from build123d import *

# Parameters (mm, degrees)
BOSS_EXTRUDE1_DEPTH = 88.9
CUT_EXTRUDE1_DEPTH  = 102.108


with BuildPart() as part:
    # Sketch2 → Boss-Extrude1 (new body)
    with BuildSketch(Plane(origin=(0, 0, 0), x_dir=(1, 0, 0), z_dir=(0, 1, 0))):
        Polygon((-63.761896162, 30.891565806), (75.945697976, 30.891565806), (75.945697976, -58.008434194), (-29.241124355, -56.925429588), (-29.241124355, -12.83474515), (-63.761896162, -12.83474515), align=None)
        Polygon((-61.729896162, -10.80274515), (-61.729896162, 28.859565806), (73.913697976, 28.859565806), (73.913697976, -55.955405), (-27.209124355, -54.91424338), (-27.209124355, -10.80274515), align=None, mode=Mode.SUBTRACT)
    extrude(amount=BOSS_EXTRUDE1_DEPTH)

    # Sketch3 → Cut-Extrude1 (cut)
    with BuildSketch(Plane(origin=(0, 0, -30.891565806), x_dir=(-1, 0, 0), z_dir=(0, 0, -1))):
        Polygon((-75.945697976, 69.85), (-6.088103838, 88.9), (63.761896162, 69.874738021), (86.047504552, 68.33004544), (86.047504552, 107.907647221), (-94.439058548, 107.907647221), (-94.439058548, 69.85), align=None)
    extrude(amount=-CUT_EXTRUDE1_DEPTH, mode=Mode.SUBTRACT)


solid = part.part
Could you check a few things on this model? Use its own coordinates, in mm. A direction names the side the tool comes from. Give positions to 0.01 mm unless a question says otherwise; leave off trailing zeros. Order: outer loops, then holes, each group sorted by start corner. A loop starts at its lowest first (then second) coordinate and runs counter-clockwise, first axis right, second up.
Item 1: For faces 5 (the face through (-29.241, 39, 35)), 6 (the face through (11.6, 0, -29.5)), 7 (the face through (-44, 39, 10.803)), which set-ups out of +Z, -Z, +X, -X, +Y, -Y let a thin tool reach every point of the face, with its end or its side?
Item 2: If we section it at A-A, the plane z = 24.5: Write out the boundary of the cut face in (x, y), plus the area to 3 significant figures.
Item 3: I need wall thicknesses on line 1 (Z direction, x = -34, y = 4); line 2 (X direction, y = 53, z = -12); line 3 (X direction, y = 18, z = 38.5). Which ranges of each line are inside material? Lowest first, please.
Item 4: If we section it at C-C, the plane y = 26: Write out the boundary of the cut face in (x, z).
Item 5: I'm going to push flat-ended pins straight in: pin 1 (8 mm diameter, centred on x = -41, y = 23.5, fed in from +Z); pin 2 (4 mm diameter, centred on x = 18, y = 53, fed in from +Z); pin 3 (5 mm diameter, centred on x = 32.5, y = 43, fed in from +Z). Where does each tip first touch, or does it pass through?
Item 6: If we mould it in two halves opening along Z, with no side actions, what happens to faces 1 (the face through (5, 44, -28.86)), 2 (the face through (-61.73, 35, -9)), 3 (the face through (75.946, 34, 13)), 4 (the face through (5, 44, -30.892))? For each: pulls with the +Z half, pulls with the -Z half, needs draft (parallel to the pull), parting line crosses it, or undercut.
Item 7: If we section it at B-B, the plane x = 17.5: Write out the boundary of the cut face in (y, z), plus the area to 3 significant figures.
Values:
1. face 5: +Z, -X, +Y, -Y
1. face 6: +Z, -Z, +X, -X, -Y
1. face 7: +Y, -Y
2. outline: (-29.24, 0) - (-27.21, 0) - (-27.21, 79.83) - (-29.24, 79.28) - close; (73.91, 0) - (75.95, 0) - (75.95, 69.85) - (73.91, 70.4) - close
2. area: 304 mm2
3. line 1: z = -30.89 to -28.86, 10.8 to 12.83
3. line 2: x = -63.76 to -61.73, 73.91 to 75.95
3. line 3: x = -29.24 to -27.21, 73.91 to 75.95
4. outline: (-63.76, -30.89) - (75.95, -30.89) - (75.95, 58.01) - (-29.24, 56.93) - (-29.24, 12.83) - (-63.76, 12.83) - close; hole (-61.73, -28.86) - (73.91, -28.86) - (73.91, 55.96) - (-27.21, 54.91) - (-27.21, 10.8) - (-61.73, 10.8) - close
5. pin 1: stops at z = 12.83
5. pin 2: stops at z = 57.43
5. pin 3: stops at z = 57.59
6. face 1: undercut
6. face 2: undercut
6. face 3: needs draft
6. face 4: pulls with the -Z half
7. outline: (0, -30.89) - (85.79, -30.89) - (85.79, -28.86) - (0, -28.86) - close; (0, 55.37) - (85.79, 55.37) - (85.79, 57.41) - (0, 57.41) - close
7. area: 349 mm2
